Verification items for this drawing (mm, ordinates from the low corner). Give positions to 0.01 mm unless a question says otherwise; leave off trailing zeros. Loops run counter-clockwise (first coordinate to the right, second up) from the corner with the lowest first, then second, coordinate; pieces in that order, holes last. Notation, with made-up numbers: (27.25, 40.25) -> (80.25, 40.25) arc R6 ccw to (80.25, 49.25) -> close; hole circle Ø11 at (25.25, 61). An arc over 180 degrees is marked (long way). Answer as a JSON object with one key per item and string values.
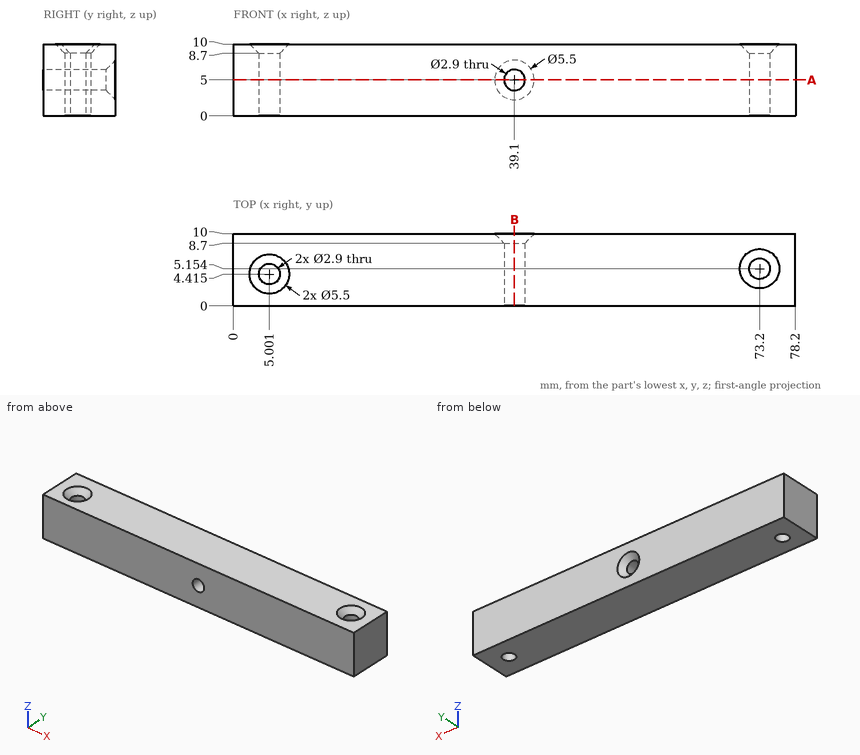
1) Section check B-B on x = 39.1. Record the cut outline in (y, z).
Geometry check:
{"outline": "(0, 0) -> (10, 0) -> (10, 2.25) -> (8.7, 3.55) -> (0, 3.55) -> close; (0, 6.45) -> (8.7, 6.45) -> (10, 7.75) -> (10, 10) -> (0, 10) -> close"}
2) Material ranges on line 1 along X through (y, z) = (4.25, 1.25) (1 decimal); line 2 along Y through (x, z) = (73.2, 4) (1 decimal); line 3 along Z through (x, y) = (39.1, 4), recorded low to high. Write a range as from..to.
Geometry check:
{"line 1": "x = 0..3.6, 6.4..72.1, 74.3..78.2", "line 2": "y = 0..3.7, 6.6..10", "line 3": "z = 0..3.55, 6.45..10"}
3) Depth check by flat-ended pin: P1, Ø3.5, axis at x = 5, y = 4.41, coming from the +Z side (1 decimal). Enter the tip coordinate at first touch or a pass-through.
Geometry check:
{"P1": "stops at z = 9"}
4) Section check A-A on z = 5. Count the separate pieces of the cut face and the enclosed holes in it, plus the area to 3 significant figures.
Geometry check:
{"separate pieces": "2", "enclosed holes": "2", "area": "738 mm2"}
